Could you check a few things on this model? Use its own coordinates, in mm. A direction names the side the tool comes from. Round coordinates to 2 decimals unless told otherwise and drop trailing zeros. Loops run counter-clockwise (first coordinate to the right, second up) from the corner with the lowest first, then second, coordinate; pieces in that order, holes last. Notation, with made-up numbers: M 22.25,50 L 35.25,50 A12 ccw 35.25,57 Z; hole C 17.5,45 d8. An arc over 180 degrees is marked long. Return JSON: item names as keys, results as strings. Group by question number.
```python
from build123d import *

# Parameters (mm, degrees)
EXTRUDE_1_DEPTH          = 45
SHELL_11_T               = -1
CUT_EXTRUDE_3_DEPTH      = 54.711648372
CUT_EXTRUDE_3_DEPTH_BACK = 54.711648372
CUT_EXTRUDE_5_DEPTH      = 58.757607161
CUT_EXTRUDE_5_DEPTH_BACK = 58.757607161
SKETCH_3_R               = 2.5
EXTRUDE_START            = 2
SKETCH_5_R               = 15
EXTRUDE_4_DEPTH          = 2
FILLET_5_R               = 2
CUT_EXTRUDE_6_DEPTH      = 56.398025084
CUT_EXTRUDE_6_DEPTH_BACK = 56.398025084
SKETCH_6_R               = 5
FILLET_6_R               = 2
FILLET_7_R               = 2


with BuildPart() as part:
    # 草图1 → 凸台-拉伸1 (new body)
    with BuildSketch(Plane.XY):
        with BuildLine():
            Line((10.198039027, -11), (25.198039027, -11))
            Line((25.198039027, -11), (25.198039027, 11))
            Line((25.198039027, 11), (10.198039027, 11))
            ThreePointArc((10.198039027, 11), (-15, 0), (10.198039027, -11))
        make_face()
    extrude(amount=EXTRUDE_1_DEPTH)

    # 抽壳11
    shell_11_openings = [part.faces().sort_by_distance(p)[0] for p in [
        (5.138978192, 0, 45),
        (5.138978192, 0, 0),
        (25.198039027, 0, 22.5),
    ]]
    offset(amount=SHELL_11_T, openings=shell_11_openings, kind=Kind.INTERSECTION)

    # 草图2 → 切除-拉伸3 (cut, two sides: drawn at the far end of the back side and taken through both)
    with BuildSketch(Plane(origin=(0, 0, 0), x_dir=(1, 0, 0), z_dir=(0, 1, 0)).offset(-CUT_EXTRUDE_3_DEPTH_BACK)):
        with BuildLine():
            Line((10.198039027, -45), (-4.526158017, -12.089687708))
            ThreePointArc((-4.526158017, -12.089687708), (-8.753229506, -7.052958097), (-15, -5))
            Line((-15, -5), (-15, -45))
            Line((-15, -45), (10.198039027, -45))
        make_face()
    extrude(amount=CUT_EXTRUDE_3_DEPTH + CUT_EXTRUDE_3_DEPTH_BACK, mode=Mode.SUBTRACT)

    # 草图3 → 切除-拉伸5 (cut, two sides: drawn at the far end of the back side and taken through both)
    with BuildSketch(Plane(origin=(0, 11, 0), x_dir=(1, 0, 0), z_dir=(0, 1, 0)).offset(-CUT_EXTRUDE_5_DEPTH_BACK)):
        with Locations(Location((17.698039027, -38, 0), (0, 0, 270))):
            Circle(SKETCH_3_R)
    extrude(amount=CUT_EXTRUDE_5_DEPTH + CUT_EXTRUDE_5_DEPTH_BACK, mode=Mode.SUBTRACT)

    # 草图5 → 凸台-拉伸4 (add)
    with BuildSketch(Plane(origin=(0, 0, 0), x_dir=(-1, 0, 0), z_dir=(0, 0, -1)).offset(EXTRUDE_START)):
        Circle(SKETCH_5_R)
    extrude(amount=-EXTRUDE_4_DEPTH)

    # 圆角5
    # the kernel refuses this fillet: 2 mm, written as the material it takes off along each edge
    with BuildSketch(Plane(origin=(0, 0, -2), x_dir=(-1, 0, 0), z_dir=(0, -1, 0))) as fillet_5_piece_1:
        with BuildLine():
            CenterArc((15 - FILLET_5_R, -FILLET_5_R), FILLET_5_R, 0, 90)
            Line((15 - FILLET_5_R, 0), (15, 0))
            Line((15, 0), (15, -FILLET_5_R))
        make_face()
    revolve(axis=Axis((0, 0, -2), (0, 0, -1)), mode=Mode.SUBTRACT)

    # 草图6 → 切除-拉伸6 (cut, two sides: drawn at the far end of the back side and taken through both)
    with BuildSketch(Plane(origin=(0, 0, -2), x_dir=(-1, 0, 0), z_dir=(0, 0, -1)).offset(-CUT_EXTRUDE_6_DEPTH_BACK)):
        Circle(SKETCH_6_R)
    extrude(amount=CUT_EXTRUDE_6_DEPTH + CUT_EXTRUDE_6_DEPTH_BACK, mode=Mode.SUBTRACT)

    # 圆角6
    fillet_6_edges = [part.edges().sort_by_distance(p)[0] for p in [
        (25.198039027, 10.5, 0),
        (25.198039027, 10.5, 45),
    ]]
    fillet(fillet_6_edges, radius=FILLET_6_R)

    # 圆角7
    fillet_7_edges = [part.edges().sort_by_distance(p)[0] for p in [
        (10.198039027, -10.5, 45),
        (10.198039027, 10.5, 45),
        (25.198039027, -10.5, 0),
        (25.198039027, -10.5, 45),
    ]]
    fillet(fillet_7_edges, radius=FILLET_7_R)


solid = part.part
```
1. On a 3-axis mill with a long thin cutter (end or side, diameter ignored), from which of +Z, -Z, +X, -X, +Y, -Y can I reach the whole of each face in a straight line? I mean faces 4 (the face through (-6, 0, 0)), 5 (the face through (24.597, -10.493, 44.43)), 6 (the face through (18, -11, 22)), 7 (the face through (3.13, 13.82, 29.2)), 8 (the face through (18, 11, 22)). Say none if no direction works.
2. If we section it at C-C, the plane x = 0: Please give me the cut outline in (y, z).
3. If we section it at B-B, the plane z = 17.5: Please give me the cut outline in (x, y), then the cut area to 3 significant figures.
4. We'd pull the mould along Y, two halves only. Please class faces 1 (the face through (24.628, 10.507, 44.399)), 2 (the face through (7.48, -13, 12.06)), 3 (the face through (7.29, 11.95, 11.93)): +Y half, -Y half, draft (parallel to the pull), parting line (faces both ways), or undercut.
5. I need wall thicknesses on probe 1 along Y at (x, z) = (22.5, 15.5); probe 2 along Y at (x, z) = (0, 10); probe 3 along X at (y, z) = (12.5, 9). Which ranges of each line are inside material? Lowest first, please.
6. I'm going to push flat-ended pins straight in: pin 1 Ø7.5 at (x, z) = (19, 30.5) entering from -Y; pin 2 Ø3 at (x, z) = (6, 13.5) entering from -Y; pin 3 Ø6 at (x, z) = (-4, 13) entering from -Y. Where does each tip first touch, or does it pass through?
7. If we section it at A-A, the plane y = 0: Please give me the cut outline in (x, z), then the cut area to 3 significant figures.
8. If we section it at D-D, the plane z = 38: Please give me the cut outline in (x, y).
Geometry results:
{
 "1": {"face 4": "+Z", "face 5": "+Z, +X, +Y, -Y", "face 6": "+Z, -Z, +X, -Y", "face 7": "+Z, -X, +Y, -Y", "face 8": "+Z, -Z, +X, +Y"},
 "2": {"outline": "M -15,0 A2 ccw -13,-2 L -5,-2 L -5,0 L -14,0 L -14,22.21 L -15,22.21 Z; M 5,-2 L 13,-2 A2 ccw 15,0 L 15,22.21 L 14,22.21 L 14,0 L 5,0 Z"},
 "3": {"outline": "M -2.11,-14.85 A15 ccw 10.2,-11 L 25.2,-11 L 25.2,-10 L 9.8,-10 A14 cw -2.11,-13.84 Z; M -2.11,13.84 A14 cw 9.8,10 L 25.2,10 L 25.2,11 L 10.2,11 A15 ccw -2.11,14.85 Z", "area": "56.7 mm^2"},
 "4": {"face 1": "draft", "face 2": "parting line", "face 3": "undercut"},
 "5": {"probe 1": "-11 to -10, 10 to 11", "probe 2": "-15 to -14, 14 to 15", "probe 3": "-6.53 to -6.3, 6.3 to 8.29"},
 "6": {"pin 1": "y = -11", "pin 2": "y = -14.31", "pin 3": "y = -14.97"},
 "7": {"outline": "M -15,0 A2 ccw -13,-2 L -5,-2 L -5,0 L -14,0 L -14,5.08 A12 cw -15,5 Z; M 5,-2 L 13,-2 A2 ccw 15,0 L 5,0 Z", "area": "43.3 mm^2"},
 "8": {"outline": "M 7.07,-13.23 A15 ccw 10.2,-11 L 15.2,-11 L 15.2,-10 L 9.8,-10 A14 cw 7.07,-12.09 Z; M 7.07,12.09 A14 cw 9.8,10 L 15.2,10 L 15.2,11 L 10.2,11 A15 ccw 7.07,13.23 Z; M 20.2,-11 L 25.2,-11 L 25.2,-10 L 20.2,-10 Z; M 20.2,10 L 25.2,10 L 25.2,11 L 20.2,11 Z"}
}
